Could you check a few things on this drawing? It's one solid part, dimensions in mm from its lowest x, y, z. A direction names the side the tool comes from. Give positions to 0.01 mm unless a question says otherwise; leave off trailing zeros. Order: outer loops, then holes, each group sorted by start corner. A loop starts at its lowest first (then second) coordinate and runs counter-clockwise, first axis right, second up. Notation, with made-up numbers: (-15.5, -32.75) - (31.5, -32.75) arc R5 cw to (31.5, -24.75) - close; hole circle Ø9 at (64, 37.5). An arc over 180 degrees is marked (long way). Answer as CSV lines item,"result".
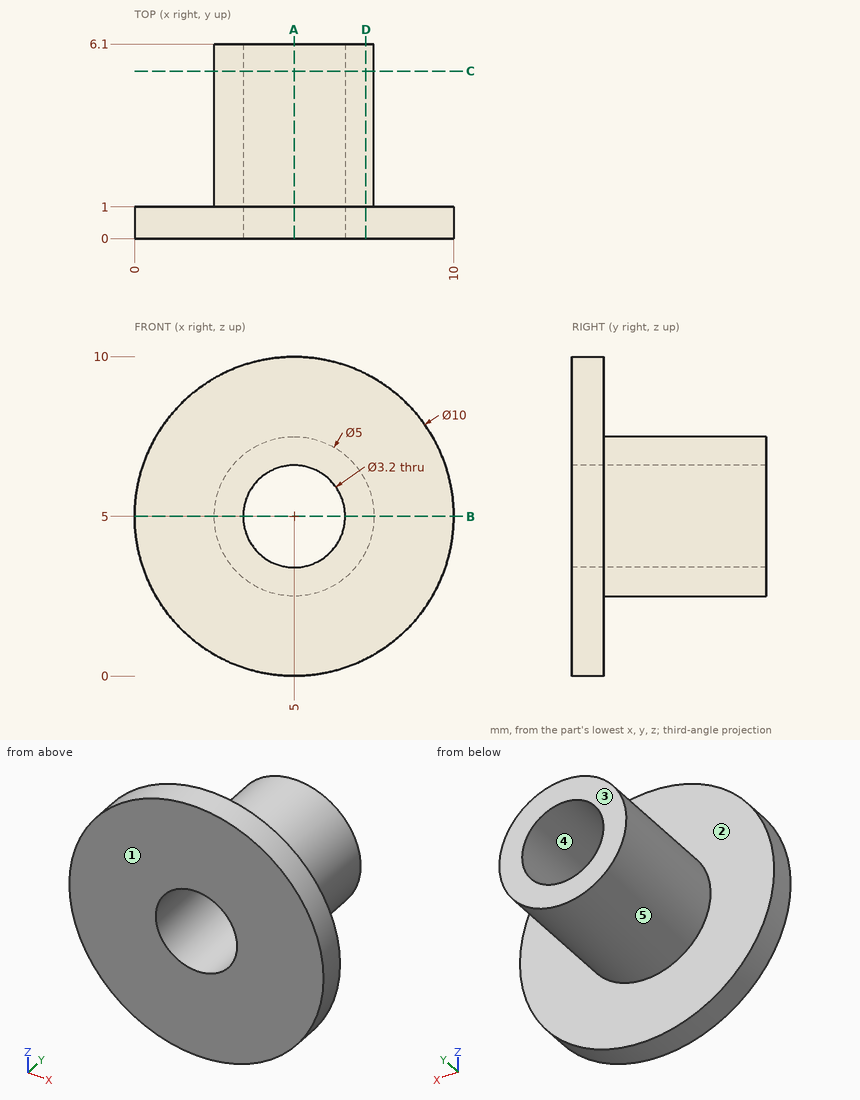
1) I'm going to push flat-ended pins straight in: P1, Ø3, axis at y = 1.5, z = 3, coming from the +X side; P2, Ø3.5, axis at x = 5, z = 5, coming from the -Y side; P3, Ø3, axis at y = 4.5, z = 8, coming from the -X side; P4, Ø3, axis at x = 3, y = 1.5, coming from the +Z side. Where does each tip first touch, or does it pass through?
Answer block:
P1,"x = 9.97"
P2,"y = 0"
P3,"x = 3"
P4,"z = 9.97"
2) I want a section at C-C on y = 5.25. Write out the boundary of the cut face in (x, z).
Answer block:
outline,"circle Ø5 at (5, 5); hole circle Ø3.2 at (5, 5)"
3) If we mould it in two halves opening along X, with no side actions, what happens to the marked faces 3, 4 and 5? For each: +X half, -X half, draft (parallel to the pull), parting line (faces both ways), or undercut.
Answer block:
face 3,"draft"
face 4,"undercut"
face 5,"parting line"
4) I want a section at A-A on x = 5. Write out the boundary of the cut face in (y, z).
Answer block:
outline,"(0, 0) - (1, 0) - (1, 2.5) - (6.1, 2.5) - (6.1, 3.4) - (0, 3.4) - close; (0, 6.6) - (6.1, 6.6) - (6.1, 7.5) - (1, 7.5) - (1, 10) - (0, 10) - close"
5) I need wall thicknesses on line 1 along Y through (x, z) = (2.75, 2.25); line 2 along X through (y, z) = (5.5, 6); line 3 along X through (y, z) = (1.75, 3). Which ranges of each line are inside material? Lowest first, please. Write a range as [from, to].
Answer block:
line 1,"[0, 1]"
line 2,"[2.71, 3.75], [6.25, 7.29]"
line 3,"[3.5, 6.5]"
6) I want a section at B-B on z = 5. Write out the boundary of the cut face in (x, y).
Answer block:
outline,"(0, 0) - (3.4, 0) - (3.4, 6.1) - (2.5, 6.1) - (2.5, 1) - (0, 1) - close; (6.6, 0) - (10, 0) - (10, 1) - (7.5, 1) - (7.5, 6.1) - (6.6, 6.1) - close"
7) I want a section at D-D on x = 7.25. Write out the boundary of the cut face in (y, z), plus the area to 3 significant figures.
Answer block:
outline,"(0, 0.53) - (1, 0.53) - (1, 3.91) - (6.1, 3.91) - (6.1, 6.09) - (1, 6.09) - (1, 9.47) - (0, 9.47) - close"
area,"20.0 mm2"
8) Which directions (+Z, -Z, +X, -X, +Y, -Y) give clear straight access to the entire face, cutting with the end or side of a thin tool? Please do the marked faces 1 and 2.
Answer block:
face 1,"+Z, -Z, +X, -X, -Y"
face 2,"+Y"
